Part model, mm, in its own coordinate system. A direction names the side the tool comes from. Round coordinates to 2 decimals unless told otherwise and drop trailing zeros. Loops run counter-clockwise (first coordinate to the right, second up) from the corner with the lowest first, then second, coordinate; pieces in that order, holes last. Notation, with made-up numbers: (7.25, -34.75) - (18.25, -34.75) arc R22 cw to (18.25, -3.75) - close; hole circle Ø6 at (1.5, 77.5). An arc over 180 degrees is marked (long way). Put each result on its own line as item: value.
from build123d import *

# Parameters (mm, degrees)
F0_R     = 127
F0_R_2   = 165.1
F1_DEPTH = 254


# Not quite as in the source:
# - ends of sketch curves that miss each other by under 0.0002 mm in the source are joined


with BuildPart() as f1:
    # F0 (on Front) → F1 (new body)
    with BuildSketch(Plane.XZ):
        with BuildLine():
            Line((1314.5506856, -451.7077834), (1466.9506856, -299.3077834))
            Line((1466.9506856, -299.3077834), (1466.9506856, -71.2509878))
            Line((1466.9506856, -71.2509878), (1314.5506856, 81.1490122))
            Line((1314.5506856, 81.1490122), (-57.0493144, 325.4681832))
            Line((-57.0493144, 325.4681832), (-184.0493144, 198.4681832))
            Line((-184.0493144, 198.4681832), (-184.0493144, 46.0681832))
            Line((-184.0493144, 46.0681832), (-91.0235416, -153.4262362))
            ThreePointArc((-91.0235416, -153.4262362), (-112.5228808858, -205.3302952862), (-162.3556290296, -179.3889979113))
            Line((-162.3556290296, -179.3889979113), (-742.8493144, -334.9318168))
            Line((-742.8493144, -334.9318168), (-488.8493144, -588.9318168))
            Line((-488.8493144, -588.9318168), (196.9506856, -588.9318168))
            Line((196.9506856, -588.9318168), (1314.5506856, -451.7077834))
        make_face()
        with Locations((1238.3506856, -182.5318168)):
            Circle(F0_R, mode=Mode.SUBTRACT)
        with Locations((69.9506856, 46.0681832)):
            Circle(F0_R_2, mode=Mode.SUBTRACT)
    extrude(amount=F1_DEPTH)


solid = f1.part
1. Tool access for faces 1 (the flat face through (-184.049, -125, 123)), 2 (the flat face through (1391.8, -125.2, 3.9)), 3 (the flat face through (-138.19, -125.22, -52.28)): list every direction of +Z, -Z, +X, -X, +Y, -Y with a clear straight run to the whole face (end or side of a thin tool).
A:
face 1: +Z, -X, +Y, -Y
face 2: +Z, +X, +Y, -Y
face 3: -X, +Y, -Y
2. Band-saw the part on B-B (z = 169.5). List the corners of the cut face in (x, y).
A:
outline: (-184.05, -254) - (-39.7, -254) - (-39.7, 0) - (-184.05, 0) - close; (179.6, -254) - (818.55, -254) - (818.55, 0) - (179.6, 0) - close
3. Probe line 1 along Z through (x, y) = (-59.5, -216.5); line 2 along X through (y, z) = (-203, -129); line 3 along Z through (x, y) = (26, -146). List the from-to ranges inside material, lowest first. Write a range as [from, to].
A:
line 1: z = [-588.93, -56.4], [148.54, 323.02]
line 2: x = [-102.41, 1123.18], [1353.52, 1466.95]
line 3: z = [-588.93, -113.07], [205.21, 310.67]
4. Band-saw the part on C-C (x = 1140). List the corners of the cut face in (y, z), plus the area to 3 significant figures.
A:
outline: (-254, -473.14) - (0, -473.14) - (0, -262.88) - (-254, -262.88) - close; (-254, -102.18) - (0, -102.18) - (0, 112.24) - (-254, 112.24) - close
area: 108,000 mm²
5. Band-saw the part on D-D (y = -118.5). List the corners of the cut face in (x, z), plus the area to 3 significant figures.
A:
outline: (-742.85, -334.93) - (-488.85, -588.93) - (196.95, -588.93) - (1314.55, -451.71) - (1466.95, -299.31) - (1466.95, -71.25) - (1314.55, 81.15) - (-57.05, 325.47) - (-184.05, 198.47) - (-184.05, 46.07) - (-91.02, -153.43) arc R38.1 cw (long way) to (-162.36, -179.39) - close; hole circle Ø330.2 at (69.95, 46.07); hole circle Ø254 at (1238.35, -182.53)
area: 1,180,000 mm²
6. Pin check, flat tips, straight feed: P1, Ø10, axis at y = -186.5, z = 26.5, coming from the +X side; P2, Ø4, axis at x = 709, y = -46, coming from the -Z side; P3, Ø1, axis at x = 625.5, z = -454, coming from the +Y side; P4, Ø8, axis at x = 1116, y = -174, coming from the -Z side. Stop position of each tip, or through.
A:
P1: stops at x = 1374.2
P2: stops at z = -526.31
P3: stops at y = 0
P4: stops at z = -476.58
7. Two-plate mould, pull along X, no slides. Class faces 4 (the cylindrical face through (1137.57, -125.22, -259.81)), 5 (the flat face through (-448.54, -125.22, -256.07)), 6 (the flat face through (347, -254, -227)): pulls with the +X half, pulls with the -X half, needs draft (parallel to the pull), parting line crosses it, or undercut.
A:
face 4: undercut
face 5: pulls with the -X half
face 6: needs draft
8. Band-saw the part on A-A (z = -90.5). List the corners of the cut face in (x, y).
A:
outline: (-120.37, -254) - (-22.82, -254) - (-22.82, 0) - (-120.37, 0) - close; (162.73, -254) - (1150.83, -254) - (1150.83, 0) - (162.73, 0) - close; (1325.87, -254) - (1466.95, -254) - (1466.95, 0) - (1325.87, 0) - close
